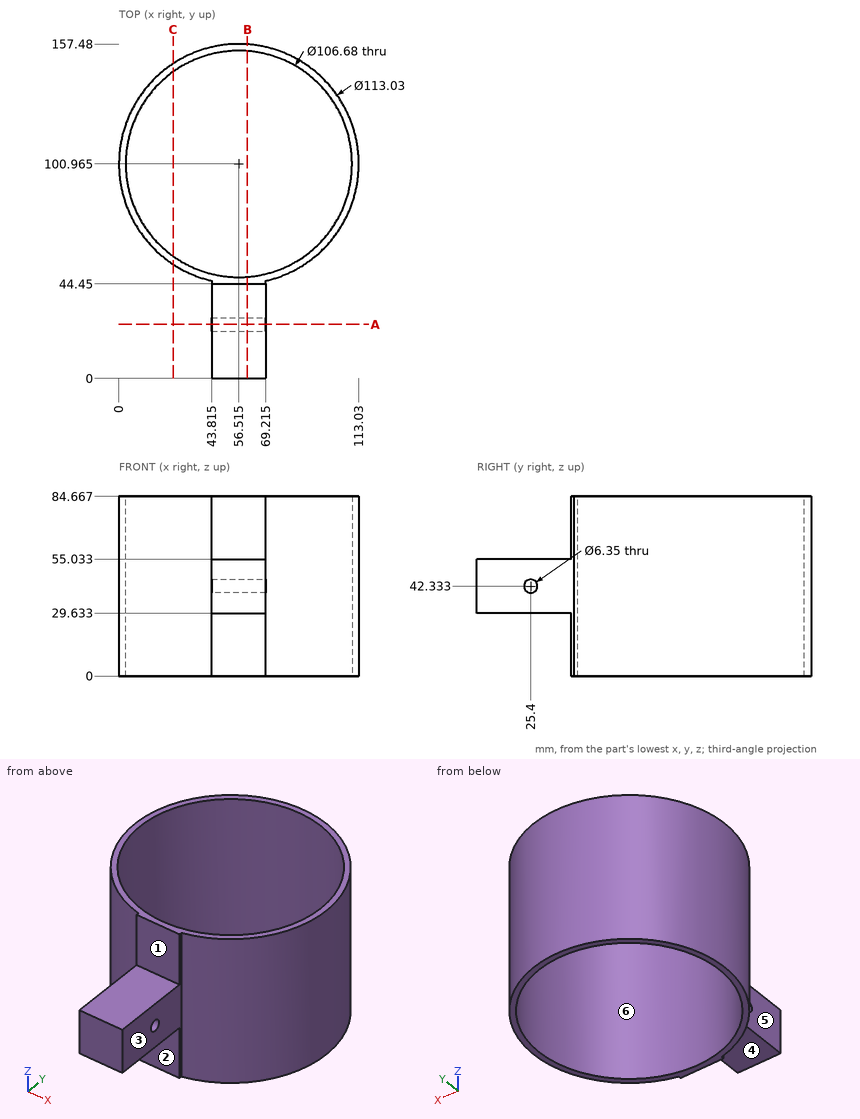
Check sheet for the drawn part. Datum: minimum x, y, z corner. Units: mm. A direction names the side the tool comes from. Coordinates: 2 decimals unless noted, no trailing zeros. Order: outer loops, then holes, each group sorted by start corner. A loop starts at its lowest first (then second) coordinate and runs counter-clockwise, first axis right, second up. Notation, with made-up numbers: M 32,3 L 43,3 A10 cw 43,12 Z; hole C 54,35.5 d3. An arc over 180 degrees is marked long. One line per question, with ' | ' between items. Start each with the question number.
Item 1: Cross-section at C-C on x = 25.5. Enter the section's corners in (y, z).
Item 2: Cross-section at B-B on x = 60.5. State how many separate pieces and enclosed holes the cut face has, then the cut area to 3 significant figures.
Item 3: Material ranges on L1, parallel to Y at x = 55.5, z = 47.5 (1 decimal); L2, parallel to X at y = 18.5, z = 44 (1 decimal); L3, parallel to Y at x = 10, z = 23.5 (1 decimal), recorded low to high. Write a range as [from, to].
Item 4: Draft check along X on the marked faces 4, 5 and 6. Enter one of: pulls with the +X half, pulls with the -X half, needs draft (parallel to the pull), parting line crosses it, or undercut.
Item 5: Gauge pin test, flat ends, axial feed: pin 1 (6 mm diameter, centred on x = 101, z = 64.5, fed in from +Y) (1 decimal); pin 2 (10 mm diameter, centred on y = 126.5, z = 43, fed in from -X); pin 3 (5 mm diameter, centred on x = 26, z = 70.5, fed in from +Y); pin 4 (10 mm diameter, centred on y = 99.5, z = 34.5, fed in from +X). Record the tip position at first contact, or that the pin passes through.
Item 6: Cross-section at A-A on y = 25.4. Enter the section's corners in (x, z) (1 decimal).
Item 7: Set-up check for the marked faces 1, 2 and 3: record each of +Z, -Z, +X, -X, +Y, -Y from which the full face is reachable in a straight line by a thin tool's end or side.
Findings:
1) outline: M 53.72,0 L 57.57,0 L 57.57,84.67 L 53.72,84.67 Z; M 144.36,0 L 148.21,0 L 148.21,84.67 L 144.36,84.67 Z
2) separate pieces: 2 | enclosed holes: 1 | area: 1,650 mm²
3) L1: y = [0, 47.6], [154.3, 157.5] | L2: x = [43.8, 69.2] | L3: y = [68.9, 74.9], [127.1, 133.1]
4) face 4: needs draft | face 5: pulls with the -X half | face 6: undercut
5) pin 1: stops at y = 139.3 | pin 2: stops at x = 3.86 | pin 3: stops at y = 150.05 | pin 4: stops at x = 113.03
6) outline: M 43.8,29.6 L 69.2,29.6 L 69.2,39.2 L 43.8,39.2 Z; M 43.8,45.5 L 69.2,45.5 L 69.2,55 L 43.8,55 Z
7) face 1: +Z, +X, -X, -Y | face 2: -Z, +X, -X, -Y | face 3: +Z, -Z, +X, -Y
